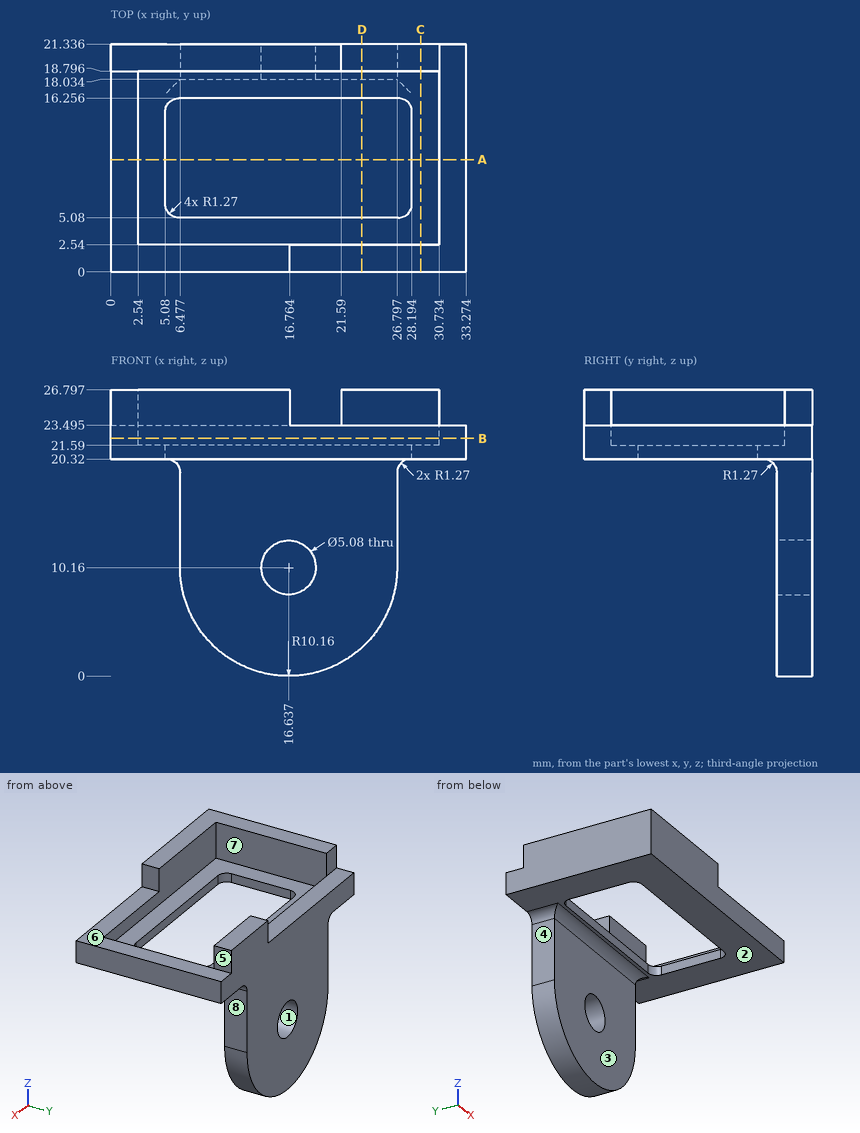
Could you check a few things on this drawing? It's one solid part, dimensions in mm from its lowest x, y, z. A direction names the side the tool comes from. Round coordinates to 2 decimals unless told otherwise and drop trailing zeros. Write each loop counter-clockwise with the first axis right and the second up, starting at its lowest first coordinate (ties: lowest second). Pieces come first, ordered by that corner, then holes. Notation, with made-up numbers: (-1, -29.75) -> (8, -29.75) arc R19 cw to (8, -15.75) -> close; hole circle Ø8 at (51.5, 36.5). An arc over 180 degrees is marked (long way). Use one line per item in the form item = value. Start each with the question number.
Q1. Which directions (+Z, -Z, +X, -X, +Y, -Y) give clear straight access to the entire face, cutting with the end or side of a thin tool? Please do the marked faces 4, 5, 6, 7 and 8.
Q2. Imagine slicing it at C-C (x = 29). Please give me the cut outline in (y, z) (3 decimals), then the cut area to 3 significant figures.
Q3. Imagine slicing it at D-D (x = 23.5). Please give me the cut outline in (y, z) (3 decimals), then the cut area to 3 significant figures.
Q4. If I drill on probe 1 along Y at (x, z) = (17, 22); probe 2 along X at (y, z) = (19.2, 10.16); probe 3 along Y at (x, z) = (13, 8.75), over which ranges is the centre line in solid material (lowest first)? Write a range as [from, to].
Q5. We'd pull the mould along Z, two halves only. Please class the marked faces 1, 2 and 3: +Z half, -Z half, draft (parallel to the pull), parting line (faces both ways), or undercut.
Q6. Imagine slicing it at B-B (z = 22.25). Please give me the cut outline in (x, y), then the cut area to 3 significant figures.
Q7. I'm going to push flat-ended pins straight in: P1, Ø4, axis at x = 9, z = 17.5, coming from the -Y side; P2, Ø0.8, axis at y = 1.5, z = 25.5, coming from the +X side; P3, Ø0.8, axis at y = 19.5, z = 25, coming from the +X side. Where does each tip first touch, or does it pass through?
Q8. Imagine slicing it at A-A (y = 10.5). Please give me the cut outline in (x, z) (3 decimals), then the cut area to 3 significant figures.
Worked out:
q1.face_4 = -Z, -X, +Y, -Y
q1.face_5 = +Z, +X, +Y, -Y
q1.face_6 = +Z, +X, -Y
q1.face_7 = +Z
q1.face_8 = -Z, +X, +Y, -Y
q2.outline = (0, 20.32) -> (21.336, 20.32) -> (21.336, 26.797) -> (18.796, 26.797) -> (18.796, 21.59) -> (2.54, 21.59) -> (2.54, 23.495) -> (0, 23.495) -> close
q2.area = 45.2 mm^2
q3.outline = (0, 20.32) -> (5.08, 20.32) -> (5.08, 21.59) -> (2.54, 21.59) -> (2.54, 23.495) -> (0, 23.495) -> close; (16.256, 20.32) -> (16.764, 20.32) arc R1.27 cw to (18.034, 19.05) -> (18.034, 2.668) -> (21.336, 2.668) -> (21.336, 26.797) -> (18.796, 26.797) -> (18.796, 21.59) -> (16.256, 21.59) -> close
q3.area = 89.6 mm^2
q4.probe_1 = [0, 2.54], [18.8, 21.34]
q4.probe_2 = [6.48, 14.1], [19.18, 26.8]
q4.probe_3 = [18.03, 21.34]
q5.face_1 = undercut
q5.face_2 = -Z half
q5.face_3 = draft
q6.outline = (0, 0) -> (33.27, 0) -> (33.27, 21.34) -> (0, 21.34) -> close; hole (2.54, 2.54) -> (30.73, 2.54) -> (30.73, 18.8) -> (2.54, 18.8) -> close
q6.area = 252 mm^2
q7.P1 = 17.95
q7.P2 = 16.76
q7.P3 = 30.73
q8.outline = (0, 20.32) -> (5.08, 20.32) -> (5.08, 21.59) -> (2.54, 21.59) -> (2.54, 26.797) -> (0, 26.797) -> close; (28.194, 20.32) -> (33.274, 20.32) -> (33.274, 23.495) -> (30.734, 23.495) -> (30.734, 21.59) -> (28.194, 21.59) -> close
q8.area = 31.0 mm^2
